from build123d import *

# Parameters (mm, degrees)
F0_R     = 7.990862
F1_DEPTH = 3


with BuildPart() as f1:
    # F0 (on Front) → F1 (new body)
    with BuildSketch(Plane.XZ):
        with BuildLine():
            Line((30, 25), (-30, 25))
            ThreePointArc((-30, 25), (-33.535534, 23.535534), (-35, 20))
            Line((-35, 20), (-35, -22))
            Line((-35, -22), (-21, -22))
            Line((-21, -22), (-21, -25))
            Line((-21, -25), (-13, -25))
            Line((-13, -25), (-13, -22))
            Line((-13, -22), (13, -22))
            Line((13, -22), (13, -25))
            Line((13, -25), (21, -25))
            Line((21, -25), (21, -22))
            Line((21, -22), (35, -22))
            Line((35, -22), (35, 20))
            ThreePointArc((35, 20), (33.535534, 23.535534), (30, 25))
        make_face()
        with Locations((-13, 0)):
            Circle(F0_R, mode=Mode.SUBTRACT)
        with Locations((13, 0)):
            Circle(F0_R, mode=Mode.SUBTRACT)
    extrude(amount=F1_DEPTH)


solid = f1.part
For this review, take the finished solid that the model builds, in its own axes (mm). A direction names the side the tool comes from. Round coordinates to 2 decimals unless told otherwise and drop trailing zeros. Order: outer loops, then holes, each group sorted by start corner. A loop starts at its lowest first (then second) coordinate and runs counter-clockwise, first axis right, second up. Notation, with made-up numbers: M -24.75,-7 L 23.25,-7 A14 ccw 23.25,18 Z; hole C 68,-14 d9. An arc over 180 degrees is marked long. Use a Markdown table: item, result. Add a question column.
Item 1: Tool access review of faces 5 (the flat face through (-28, -1, -22)), 6 (the flat face through (21, -1, -24)), 7 (the flat face through (0, 0, 0)), 8 (the flat face through (13, -1, -23)): name each direction out of +Z, -Z, +X, -X, +Y, -Y from which nothing blocks a thin tool from reaching the whole face with its end or side.
Item 2: To check wall thickness, follow line 1 along X through (y, z) = (-1.65, -0.5); line 2 along Z through (x, y) = (-23, -2.1); line 3 along X through (y, z) = (-0.15, -2). State the ranges of each line that lie inside material, in increasing order.
Item 3: Add section B-B, the plane x = -19. Give the boundary of the cut face in (y, z).
Item 4: Mouldability with a two-part tool opening along Z and no side actions: class faces 1 (the flat face through (0, -1, -22)), 2 (the cylindrical face through (-19.341, -1.479, -4.862)), 3 (the cylindrical face through (-33, -1, 24)), 4 (the cylindrical face through (5.017, -1.479, 0.351)) as released by +Z, released by -Z, zero draft, split by the parting line, or undercut.
Item 5: Add section A-A, the plane z = 0. Give the boundary of the cut face in (x, y), then the cut area to 3 significant figures.
Item 6: Insertion check: pin 1 (1.5 mm diameter, centred on x = 4, y = -2, fed in from -Z); pin 2 (12 mm diameter, centred on x = -27.5, z = 6, fed in from +Y); pin 3 (1.5 mm diameter, centred on y = -2, z = -23.5, fed in from -X); pin 4 (0.9 mm diameter, centred on y = -1.5, z = -23.5, fed in from +X). Each pin has a flat end and moves straight along its axis. Give the tip position at first contact, or say it passes through.
Item 7: Add section D-D, the plane x = 8. Give the boundary of the cut face in (y, z), then the cut area to 3 significant figures.
Item 8: Add section C-C, the plane x = -27. Give the boundary of the cut face in (y, z).
Geometry results:
| question | item | result |
|---|---|---|
| 1 | face 5 | -Z, -X, +Y, -Y |
| 1 | face 6 | -Z, +X, +Y, -Y |
| 1 | face 7 | +Z, -Z, +X, -X, +Y |
| 1 | face 8 | -Z, +Y, -Y |
| 2 | line 1 | x = -35 to -20.98, -5.02 to 5.02, 20.98 to 35 |
| 2 | line 2 | z = -22 to 25 |
| 2 | line 3 | x = -35 to -20.74, -5.26 to 5.26, 20.74 to 35 |
| 3 | outline | M -3,-25 L 0,-25 L 0,-5.28 L -3,-5.28 Z; M -3,5.28 L 0,5.28 L 0,25 L -3,25 Z |
| 4 | face 1 | released by -Z |
| 4 | face 2 | undercut |
| 4 | face 3 | released by +Z |
| 4 | face 4 | undercut |
| 5 | outline | M -35,-3 L -20.99,-3 L -20.99,0 L -35,0 Z; M -5.01,-3 L 5.01,-3 L 5.01,0 L -5.01,0 Z; M 20.99,-3 L 35,-3 L 35,0 L 20.99,0 Z |
| 5 | area | 114 mm² |
| 6 | pin 1 | stops at z = -22 |
| 6 | pin 2 | stops at y = 0 |
| 6 | pin 3 | stops at x = -21 |
| 6 | pin 4 | stops at x = 21 |
| 7 | outline | M -3,-22 L 0,-22 L 0,-6.23 L -3,-6.23 Z; M -3,6.23 L 0,6.23 L 0,25 L -3,25 Z |
| 7 | area | 104 mm² |
| 8 | outline | M -3,-22 L 0,-22 L 0,25 L -3,25 Z |
